Part model, mm, in its own coordinate system. A direction names the side the tool comes from. Give positions to 0.01 mm unless a question says otherwise; leave off trailing zeros. Write each loop counter-clockwise with the first axis right and the second up, starting at its lowest first coordinate (ties: lowest second). Pieces come first, ordered by that corner, then holes. Notation, with made-up numbers: M 74,17.5 L 116,17.5 A25 ccw 116,32.5 Z; hole C 73,41.5 d4. An arc over 180 degrees is marked long. Answer as CSV lines item,"result". Start each with the question number.
Item 1: 3-axis set-ups, long thin cutter, end or side, ignore diameter. For faces 1 (the flat face through (-1, 5.424, 3)), 2 (the flat face through (-4.62, -1.02, 3.79)), 3 (the flat face through (-10.1, -0.2, -6.3)), 4 (the flat face through (6, 8.869, 1)), 5 (the cylindrical face through (14.763, 6.35, 1.252)): which of +Z, -Z, +X, -X, +Y, -Y reach the whole face in a straight line?
Item 2: Band-saw the part on D-D, the plane y = 21.25. List the corners of the cut face in (x, z).
Item 3: Band-saw the part on B-B, the plane x = -23.5. List the corners of the cut face in (y, z) (3 decimals).
Item 4: Two-plate mould, pull along Z, no slides. Class faces 6 (the flat face through (9.081, 11, 3)), 7 (the flat face through (-6.583, 13.994, -8.228)), 8 (the flat face through (-24.63, 14.68, -4.73)): +Z half, -Z half, draft (parallel to the pull), parting line (faces both ways), or undercut.
Item 5: Pin check, flat tips, straight feed: pin 1 (9.5 mm diameter, centred on x = -0.5, y = 5, fed in from -Z); pin 2 (6 mm diameter, centred on x = 1.5, y = 12, fed in from +Z); pin 3 (2.5 mm diameter, centred on x = 4, z = 2.5, fed in from -Y). Stop position of each tip, or through.
Item 6: Wall check: L1, parallel to X at y = 2.25, z = 1.25; L2, parallel to Y at x = -1, z = 3.75; L3, parallel to X at y = 0.75, z = 1. Give the ranges that are in metal, low to high. Write a range as from..to.
Item 7: Band-saw the part on C-C, the plane z = 3.5. List the corners of the cut face in (x, y), then the cut area to 3 significant figures.
Item 8: Band-saw the part on A-A, the plane z = -0.75. List the corners of the cut face in (x, y), then the cut area to 3 significant figures.
from build123d import *
from build123d.topology import SkipClean

# Parameters (mm, degrees)
BOSS_EXTRUDE1_DEPTH      = 5.08
CUT_EXTRUDE1_DEPTH       = 2.54
SKETCH3_W                = 9.11222741
SKETCH3_H                = 2.54
BOSS_EXTRUDE2_DEPTH      = 5.08
BOSS_EXTRUDE3_DEPTH      = 17.78
CUT_EXTRUDE2_DEPTH       = 15.24
CUT_EXTRUDE3_DEPTH       = 11.43
CHAMFER1_SIZE            = 10.265287786
CHAMFER1_SIZE_2          = 17.78
SKETCH7_W                = 3.81
SKETCH7_H                = 3.81
CUT_EXTRUDE4_DEPTH       = 25.4
SKETCH8_W                = 6.35
SKETCH8_H                = 6.35
CUT_EXTRUDE5_DEPTH       = 2.54
BOSS_EXTRUDE4_DEPTH      = 2.54
BOSS_EXTRUDE4_DEPTH_BACK = 2.54
BOSS_EXTRUDE5_START      = -5.08
BOSS_EXTRUDE5_DEPTH      = 5.08
BOSS_EXTRUDE6_START      = -2.54
BOSS_EXTRUDE6_DEPTH      = 2.54
CUT_EXTRUDE6_DEPTH       = 55.88
CUT_EXTRUDE7_START       = -5.08
CUT_EXTRUDE7_DEPTH       = 5.08
BOSS_EXTRUDE7_DEPTH      = 2.54


# Read off the part's stored shape, not the designer's step: Boss-Extrude5, Cut-Extrude7
with BuildPart() as part:
    # Sketch1 → Boss-Extrude1 (new body)
    with BuildSketch(Plane.XY):
        with BuildLine():
            Line((8.309836615, 7.848026213), (-11.143288506, -2.544016758))
            ThreePointArc((-11.143288506, -2.544016758), (-5.385698811, 10.08162429), (8.309836615, 7.848026213))
        make_face()
    extrude(amount=BOSS_EXTRUDE1_DEPTH)

    # Sketch2 → Cut-Extrude1 (cut)
    with SkipClean():  # the faces are left unmerged after this step: merging them gives an invalid solid
        with BuildSketch(Plane(origin=(0, 0, 0), x_dir=(-1, 0, 0), z_dir=(0, 0, -1))):
            with BuildLine():
                ThreePointArc((-3.514271346, 8.165904537), (4.188876853, 7.841263336), (8.741367154, 1.618826824))
                Line((8.741367154, 1.618826824), (-3.514271346, 8.165904537))
            make_face()
            with BuildLine():
                Line((8.741367154, 1.618826824), (-3.514271346, 8.165904537))
                ThreePointArc((-3.514271346, 8.165904537), (-4.803100251, 7.480797282), (-5.962452981, 6.594031729))
                Line((-5.962452981, 6.594031729), (8.795904873, -1.290022275))
                ThreePointArc((8.795904873, -1.290022275), (8.8884379, 0.166648428), (8.741367154, 1.618826824))
            make_face()
        extrude(amount=-CUT_EXTRUDE1_DEPTH, mode=Mode.SUBTRACT)

    # Sketch3 → Boss-Extrude2 (add)
    with SkipClean():  # the faces are left unmerged after this step: merging them gives an invalid solid
        with BuildSketch(Plane(origin=(-1.416725946, 2.652004727, 0), x_dir=(0.8820318713627303, 0.4711897472360366, 0), z_dir=(0.47118974723603657, -0.8820318713627302, 0))):
            with Locations((0, 3.81)):
                Rectangle(SKETCH3_W, SKETCH3_H)
        extrude(amount=BOSS_EXTRUDE2_DEPTH)

    # Sketch4 → Boss-Extrude3 (add)
    with SkipClean():  # the faces are left unmerged after this step: merging them gives an invalid solid
        with BuildSketch(Plane.XY.offset(5.08)):
            Polygon((-2.901644401, 16.029554576), (-20.315117145, 23.754414899), (-28.34897188, 5.644403245), (-10.935499136, -2.080457077), align=None)
        extrude(amount=-BOSS_EXTRUDE3_DEPTH)

    # Sketch5 → Cut-Extrude2 (cut)
    with BuildSketch(Plane(origin=(0, 0, -12.7), x_dir=(-1, 0, 0), z_dir=(0, 0, -1))):
        Polygon((8.432077676, 13.898059844), (0.608597096, 10.427454319), (5.243513289, -0.020629328), (13.066993869, 3.449976197), (22.818538605, 7.775897978), (18.183622412, 18.223981624), align=None)
    extrude(amount=-CUT_EXTRUDE2_DEPTH, mode=Mode.SUBTRACT)

    # Sketch6 → Cut-Extrude3 (cut)
    with BuildSketch(Plane(origin=(-0.869857896, -1.960844097, 0), x_dir=(0.914093057420647, -0.4055044788598195, 0), z_dir=(0.4055044788598195, 0.914093057420647, 0))):
        Polygon((-24.011429177, -2.54), (-38.355843434, 12.7), (-24.011429177, 12.7), align=None)
    extrude(amount=CUT_EXTRUDE3_DEPTH, mode=Mode.SUBTRACT)

    # Chamfer1
    # the kernel refuses this chamfer: 17.78, 10.265287786 mm, written as the material it takes off along each edge
    with BuildSketch(Plane(origin=(-1.662566122, 65.801219022, 5.08), x_dir=(-0.052920377689547264, 0.02347622050277695, -0.9983227437537927), z_dir=(-0.40550447885981916, -0.9140930574206472, 0))) as chamfer1_piece_1:
        Polygon((CHAMFER1_SIZE * 0.998322743772, CHAMFER1_SIZE * 0.0578938624038), (-CHAMFER1_SIZE_2 * 0.0578938624027, CHAMFER1_SIZE_2 * 0.998322743754), (0, 0), align=None)
    extrude(amount=111.808769435, mode=Mode.SUBTRACT)

    # Sketch7 → Cut-Extrude4 (cut)
    with BuildSketch(Plane(origin=(5.464527568, 12.318203553, 0), x_dir=(0.9140930574206471, -0.40550447885981944, 0), z_dir=(0.4055044788598195, 0.9140930574206472, 0))):
        with Locations((-13.597429177, 8.255)):
            Rectangle(SKETCH7_W, SKETCH7_H)
    extrude(amount=-CUT_EXTRUDE4_DEPTH, mode=Mode.SUBTRACT)

    # Sketch8 → Cut-Extrude5 (cut)
    with BuildSketch(Plane(origin=(5.464527568, 12.318203553, 0), x_dir=(0.9140930574206471, -0.40550447885981944, 0), z_dir=(0.4055044788598195, 0.9140930574206472, 0))):
        with Locations((-13.597429177, 8.255)):
            Rectangle(SKETCH8_W, SKETCH8_H)
    extrude(amount=-CUT_EXTRUDE5_DEPTH, mode=Mode.SUBTRACT)

    # Sketch10 → Boss-Extrude4 (add, two sides: drawn at the far end of the back side and taken through both)
    with BuildSketch(Plane(origin=(-4.392502173, 1.948575465, 8.323044218), x_dir=(0.8894427865769886, 0.10418568638497319, 0.4450133393041759), z_dir=(-0.457046528710329, 0.20275223942991202, 0.8660254037844353)).offset(-BOSS_EXTRUDE4_DEPTH_BACK)):
        Polygon((-26.934244752, 6.677804801), (-17.901786615, 24.311013357), (0.370973372, 14.950950547), (-8.661484766, -2.682258009), align=None)
    extrude(amount=BOSS_EXTRUDE4_DEPTH + BOSS_EXTRUDE4_DEPTH_BACK)

    # Boss-Extrude5 outline → Boss-Extrude5 (add)
    with BuildSketch(Plane.XY.offset(5.08).offset(BOSS_EXTRUDE5_START)):
        with BuildLine():
            Line((2.601911551, 4.798798792), (5.962452981, 6.594031729))
            ThreePointArc((5.962452981, 6.594031729), (2.56067771, 8.513226748), (-1.33537929, 8.789133186))
            Line((-1.33537929, 8.789133186), (-0.995970787, 9.554231902))
            ThreePointArc((-0.995970787, 9.554231902), (-3.936753752, 5.290676536), (-4.972191023, 0.215838758))
            Line((-4.972191023, 0.215838758), (4.804173359, 0.215838758))
            Line((4.804173359, 0.215838758), (4.995555467, 0.318076886))
            Line((4.995555467, 0.318076886), (2.601911551, 4.798798792))
        make_face()
        with BuildLine():
            ThreePointArc((1.359063718, 11.348913861), (4.156560335, 10.647436602), (6.689412036, 9.268045458))
            ThreePointArc((6.689412036, 9.268045458), (13.973263657, 7.123458233), (17.125808977, 0.215838758))
            Line((17.125808977, 0.215838758), (20.935808977, 0.215838758))
            ThreePointArc((20.935808977, 0.215838758), (14.385521725, 11.476326272), (1.359063718, 11.348913861))
        make_face()
    extrude(amount=BOSS_EXTRUDE5_DEPTH)

    # Sketch12 → Boss-Extrude6 (add)
    with BuildSketch(Plane.XY.offset(5.08).offset(BOSS_EXTRUDE6_START)):
        with BuildLine():
            ThreePointArc((17.125808977, 0.215838758), (13.973263657, 7.123458233), (6.689412036, 9.268045458))
            ThreePointArc((6.689412036, 9.268045458), (7.533158613, 8.59630277), (8.309836615, 7.848026213))
            Line((8.309836615, 7.848026213), (2.601911551, 4.798798792))
            Line((2.601911551, 4.798798792), (4.995555467, 0.318076886))
            Line((4.995555467, 0.318076886), (-2.581764519, -3.72979894))
            Line((-2.581764519, -3.72979894), (20.935808977, 0.215838758))
            Line((20.935808977, 0.215838758), (17.125808977, 0.215838758))
        make_face()
    extrude(amount=BOSS_EXTRUDE6_DEPTH)

    # Sketch13 → Cut-Extrude6 (cut)
    with BuildSketch(Plane.XY.offset(5.08)):
        Polygon((-0.455894293, -2.594139008), (-3.041719527, -3.975511244), (-3.779661608, -2.594139008), align=None)
    extrude(amount=-CUT_EXTRUDE6_DEPTH, mode=Mode.SUBTRACT)

    # Cut-Extrude7 outline → Cut-Extrude7 (cut)
    with BuildSketch(Plane(origin=(0, 0, 0), x_dir=(-1, 0, 0), z_dir=(0, 0, -1)).offset(CUT_EXTRUDE7_START)):
        with BuildLine():
            ThreePointArc((-7.17051589, 8.901044988), (-7.026535215, 8.886389823), (-6.882817494, 8.869347956))
            Line((-6.882817494, 8.869347956), (-5.6435439, 8.869347956))
            Line((-5.6435439, 8.869347956), (-5.6435439, 8.619618869))
            ThreePointArc((-5.6435439, 8.619618869), (-3.048054454, 7.409521405), (-0.984312942, 5.424106508))
            Line((-0.984312942, 5.424106508), (2.486117219, 5.424106508))
            Line((2.486117219, 5.424106508), (2.486117219, 8.869347956))
            Line((2.486117219, 8.869347956), (1.657843224, 8.869347956))
            ThreePointArc((1.657843224, 8.869347956), (1.333203623, 9.217874986), (0.995970787, 9.554231902))
            Line((0.995970787, 9.554231902), (0.608597096, 10.427454319))
            Line((0.608597096, 10.427454319), (2.328316525, 11.190345935))
            ThreePointArc((2.328316525, 11.190345935), (0.491068934, 11.41944619), (-1.359063718, 11.34891386))
            ThreePointArc((-1.359063718, 11.34891386), (-1.695483089, 11.542277864), (-2.037543, 11.725478978))
            Line((-2.037543, 11.725478978), (-9.08080046, 11.725478978))
            Line((-9.08080046, 11.725478978), (-9.08080046, 9.293556187))
            ThreePointArc((-9.08080046, 9.293556187), (-7.884268641, 9.359318505), (-6.689412036, 9.268045458))
            ThreePointArc((-6.689412036, 9.268045458), (-6.932393011, 9.087729482), (-7.17051589, 8.901044988))
        make_face()
    extrude(amount=CUT_EXTRUDE7_DEPTH, mode=Mode.SUBTRACT)

    # Sketch15 → Boss-Extrude7 (add)
    with BuildSketch(Plane(origin=(0, 0, 2.54), x_dir=(-1, 0, 0), z_dir=(0, 0, -1))):
        Polygon((-7.906818903, 8.804382246), (4.601113672, 12.198590573), (6.567709174, 7.765467415), (3.37435699, 6.448302999), align=None)
    extrude(amount=-BOSS_EXTRUDE7_DEPTH)


solid = part.part
Output:
1,face 1,"+Z, -Z"
1,face 2,"+Z, -Z, -Y"
1,face 3,"-Z, +X, -Y"
1,face 4,"-Z"
1,face 5,"-Z, -Y"
2,outline,"M -22.82,-2.99 L -21.43,-5.19 L -21.43,-12.7 L -14.67,-12.7 L -14.67,1.31 Z"
3,outline,"M 3.493,-12.7 L 8.078,-12.7 L 8.078,-6.129 L 13.443,-7.385 L 19.707,-2.986 L 3.493,0.81 Z"
4,face 6,"draft"
4,face 7,"undercut"
4,face 8,"-Z half"
5,pin 1,"z = 0"
5,pin 2,"z = 5.08"
5,pin 3,"y = -2.84"
6,L1,"-20.7..-10.36, -4.81..3.96, 16.9..20.78"
6,L2,"-3.46..-2.88, -2.59..5.42, 6.94..11.22"
6,L3,"-17.32..-8.86, -4.96..4.76, 17.11..20.92"
7,outline,"M -19.24,1.6 L -11.27,-1.93 A11.43 ccw -11.14,-2.54 L -5.44,0.51 L -3.78,-2.59 L -0.46,-2.59 L -2.58,-3.73 L 20.94,0.22 A12.95 ccw 2.04,11.73 L 9.08,11.73 L 9.08,9.29 A9.14 ccw 6.69,9.27 A11.43 cw 6.97,9.06 L -4.6,12.2 L -2.9,16.03 L -11.21,19.71 Z; hole M -2.49,5.42 L 0.98,5.42 A8.72 cw 4.04,8 L -2.49,6.63 Z"
7,area,"525 mm²"
8,outline,"M -25.97,4.59 L -10.94,-2.08 L -9.24,1.75 L -14.98,4.3 L -10.35,14.75 L -4.6,12.2 L -2.9,16.03 L -17.94,22.7 Z"
8,area,"254 mm²"
